Check sheet for the modelled part. Datum: model origin and axes. Units: mm. Round coordinates to 2 decimals unless told otherwise and drop trailing zeros. Order: outer loops, then holes, each group sorted by start corner. A loop starts at its lowest first (then second) coordinate and runs counter-clockwise, first axis right, second up.
Autodesk Inventor part; units mm, degrees
ref_plane "YZ Plane" through (0, 0, 0) normal (1, 0, 0) x (0, 1, 0)
ref_plane "XZ Plane" through (0, 0, 0) normal (0, 1, 0) x (-1, 0, 0)
ref_plane "XY Plane" through (0, 0, 0) normal (0, 0, 1) x (1, 0, 0)
sketch "Sketch1" plane through (0, 0, 0) normal (0, 0, 1) x (1, 0, 0)
  circle A0 centre (-124.2929, 102.2868) radius 4.385
  circle A1 centre (-64.2929, 102.2868) radius 4.385
  line L0 (-116.2929, 112.2868) -> (-59.2929, 112.2868)
  line L1 (-129.2929, 92.2868) -> (-59.2929, 92.2868)
  line L2 (-124.3591, 92.2868) -> (-129.2929, 92.2868)
  line L3 (-134.2929, 107.2868) -> (-134.2929, 97.2868)
  line L4 (-54.2929, 97.2868) -> (-54.2929, 107.2868)
  arc A2 (-129.2929, 112.2868) -> (-134.2929, 107.2868) centre (-129.2929, 107.2868) ccw
  arc A3 (-134.2929, 97.2868) -> (-129.2929, 92.2868) centre (-129.2929, 97.2868) ccw
  arc A4 (-59.2929, 92.2868) -> (-54.2929, 97.2868) centre (-59.2929, 97.2868) ccw
  arc A5 (-54.2929, 107.2868) -> (-59.2929, 112.2868) centre (-59.2929, 107.2868) ccw
  line L5 (-59.2929, 112.2868) -> (-72.2929, 112.2868)
  line L6 (-116.2929, 112.2868) -> (-129.2929, 112.2868)
  circle A6 centre (-114.2929, 102.2868) radius 1
  circle A7 centre (-105.2929, 102.2868) radius 1
  circle A8 centre (-74.2929, 102.2868) radius 1
  circle A9 centre (-83.2929, 102.2868) radius 1
  point P0 (-126.1429, 102.2868)
  point P1 (-79.2929, 92.2868)
  dimension "d109" = 10
  dimension "d110" = 10
  dimension "d111" = 8.77
  dimension "d112" = 8.77
  dimension "d113" = 2
  dimension "d114" = 2
  dimension "d115" = 10
  dimension "d116" = 9
  dimension "d117" = 2
  dimension "d118" = 2
  dimension "d119" = 10
  dimension "d120" = 9
  dimension "d121" = 60
  dimension "d126" = 10
  dimension "d401" = 20
extrude "Extrusion1" add sketch "Sketch1" along normal blind 1
properties part number "sketch femur 6 cm"
1) Sectioned sample at A-A on x = -128. Record the cut outline in (y, z), and give its area (3 significant figures).
2) Scan lines: line 1 (Y direction, x = -124, z = 0.6); line 2 (X direction, y = 100, z = 0.45); line 3 (X direction, y = 105.5, z = 0.55). Record each from-to range of solid material in increasing order.
3) Gauge pin test, flat end, axial feed: pin 1 (5.5 mm diameter, centred on x = -64.29, y = 102.29, fed in from -Z). Record the tip position at first contact, or that the pin passes through.
4) Draft check along Y on faces 1 (the face through (-55.72, 93.79, 0.49)), 2 (the face through (-132.87, 110.78, 0.49)), 3 (the face through (-120.1, 101, 0.5)), 4 (the face through (-83.423, 101.295, 0.493)). Enter one of: pulls with the +Y half, pulls with the -Y half, needs draft (parallel to the pull), parting line crosses it, or undercut.
5) Sectioned sample at D-D on y = 105.5. Record the cut outline in (x, z), and give its area (3 significant figures).
6) Sectioned sample at C-C on z = 0.2. Record the cut outline in (x, y) (3 decimals).
7) Sectioned sample at B-B on y = 98.75. Record the cut outline in (x, z).
Values found:
1. outline: (92.29, 0) - (99.94, 0) - (99.94, 1) - (92.29, 1) - close; (104.63, 0) - (112.29, 0) - (112.29, 1) - (104.63, 1) - close
1. area: 15.3 mm2
2. line 1: y = 92.29 to 97.91, 106.66 to 112.29
2. line 2: x = -134.29 to -128.03, -120.55 to -68.03, -60.55 to -54.29
2. line 3: x = -134.29 to -127.28, -121.31 to -67.28, -61.31 to -54.29
3. pin 1: passes through
4. face 1: pulls with the -Y half
4. face 2: pulls with the +Y half
4. face 3: undercut
4. face 4: undercut
5. outline: (-134.29, 0) - (-127.28, 0) - (-127.28, 1) - (-134.29, 1) - close; (-121.31, 0) - (-67.28, 0) - (-67.28, 1) - (-121.31, 1) - close; (-61.31, 0) - (-54.29, 0) - (-54.29, 1) - (-61.31, 1) - close
5. area: 68.1 mm2
6. outline: (-134.293, 97.287) arc R5 ccw to (-129.293, 92.287) - (-59.293, 92.287) arc R5 ccw to (-54.293, 97.287) - (-54.293, 107.287) arc R5 ccw to (-59.293, 112.287) - (-129.293, 112.287) arc R5 ccw to (-134.293, 107.287) - close; hole circle Ø8.77 at (-124.293, 102.287); hole circle Ø2 at (-114.293, 102.287); hole circle Ø2 at (-105.293, 102.287); hole circle Ø2 at (-83.293, 102.287); hole circle Ø2 at (-74.293, 102.287); hole circle Ø8.77 at (-64.293, 102.287)
7. outline: (-134.29, 0) - (-126.89, 0) - (-126.89, 1) - (-134.29, 1) - close; (-121.7, 0) - (-66.89, 0) - (-66.89, 1) - (-121.7, 1) - close; (-61.7, 0) - (-54.29, 0) - (-54.29, 1) - (-61.7, 1) - close
